Drawing for the job (mm, zero at the part's lowest x, y, z). Coordinates: 2 decimals unless noted, no trailing zeros. Write each loop counter-clockwise with the first axis right and the second up, starting at its lowest first coordinate (ties: lowest second). Pieces come first, ordered by that corner, then holes. Notation, with made-up numbers: (36.5, 55) -> (88.5, 55) arc R23 cw to (88.5, 66) -> close; hole circle Ø1 at (26, 42.5). An arc over 180 degrees is marked (long way). Answer as CSV lines item,"result".
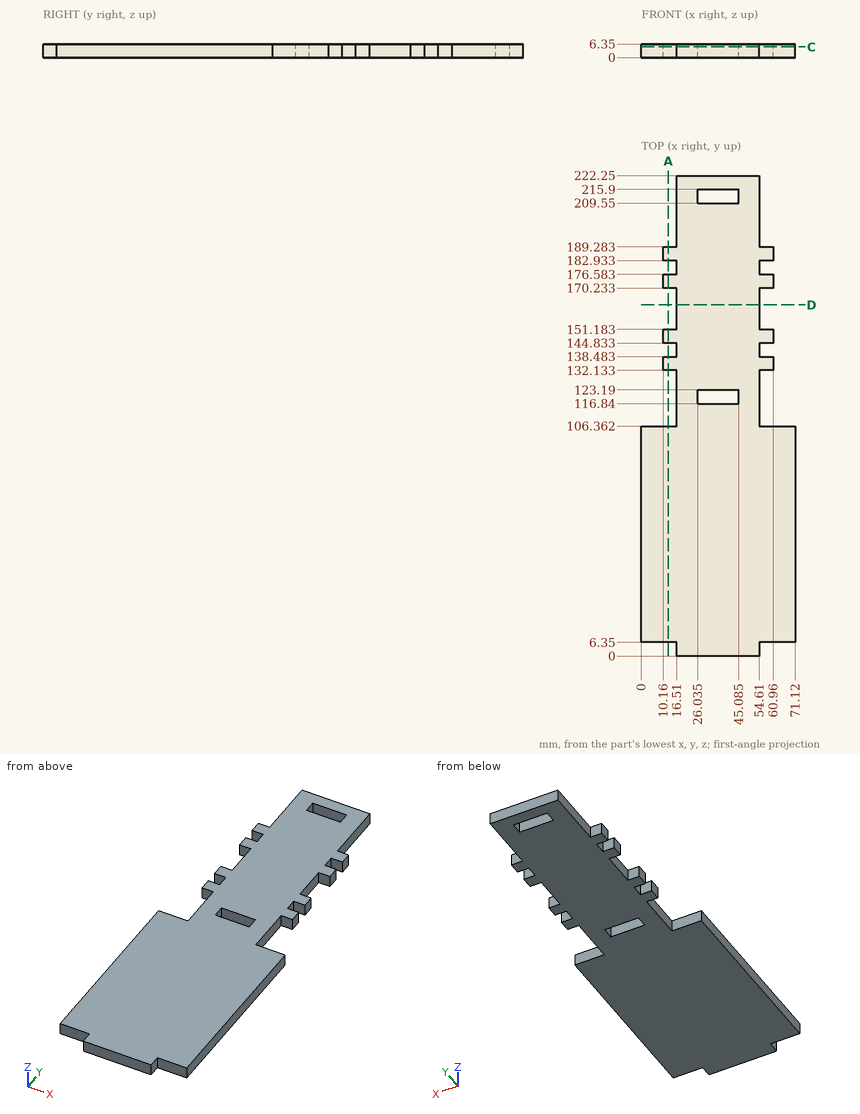
Item 1: Saw through at A-A on x = 12.5. Give the cut face in (y, z).
Answer below:
outline,"(6.35, 0) -> (106.36, 0) -> (106.36, 6.35) -> (6.35, 6.35) -> close; (132.13, 0) -> (138.48, 0) -> (138.48, 6.35) -> (132.13, 6.35) -> close; (144.83, 0) -> (151.18, 0) -> (151.18, 6.35) -> (144.83, 6.35) -> close; (170.23, 0) -> (176.58, 0) -> (176.58, 6.35) -> (170.23, 6.35) -> close; (182.93, 0) -> (189.28, 0) -> (189.28, 6.35) -> (182.93, 6.35) -> close"
Item 2: Saw through at D-D on y = 162.5. Give the cut face in (x, z), and give its area (3 significant figures).
Answer below:
outline,"(16.51, 0) -> (54.61, 0) -> (54.61, 6.35) -> (16.51, 6.35) -> close"
area,"242 mm2"
Item 3: Flat gauge pins, fed straight in: pin 1 (1.5 mm diameter, centred on x = 62.5, y = 187.5, fed in from +Z); pin 2 (1.9 mm diameter, centred on y = 159, z = 2, fed in from +X); pin 3 (3 mm diameter, centred on y = 172, z = 4.5, fed in from +X); pin 4 (1.9 mm diameter, centred on x = 58, z = 4.5, fed in from +Y). Where does each tip first touch, or does it go through?
Answer below:
pin 1,"passes through"
pin 2,"stops at x = 54.61"
pin 3,"stops at x = 60.96"
pin 4,"stops at y = 189.28"
Item 4: Saw through at C-C on z = 5. State how many separate pieces and enclosed holes the cut face has, and give its area (4 significant figures).
Answer below:
separate pieces,"1"
enclosed holes,"2"
area,"11,850 mm2"
Item 5: Wall check: line 1 (Y direction, x = 13, z = 0.5); line 2 (Y direction, x = 28, z = 2.75); line 3 (Y direction, x = 62.5, z = 3.75). Give the ranges that are in metal, low to high. Write a range as from..to.
Answer below:
line 1,"y = 6.35..106.36, 132.13..138.48, 144.83..151.18, 170.23..176.58, 182.93..189.28"
line 2,"y = 0..116.84, 123.19..209.55, 215.9..222.25"
line 3,"y = 6.35..106.36"
